```python
from build123d import *

# Parameters (mm, degrees)
F2_R     = 1.5875
F3_DEPTH = 21.717
F4_R     = 4.7625
F5_DEPTH = 9.525


with BuildPart() as f1:
    # F0 (on Front) → F1 (revolve)
    with BuildSketch(Plane.XZ):
        with BuildLine():
            Line((0, 57.6952844858), (0, 0))
            Line((0, 0), (7.62, 0))
            Line((7.62, 0), (7.62, 5.334))
            add(Edge.make_bspline(
                [(7.62, 5.334), (10.5113989407, 7.1572880683), (17.4669983954, 11.2866916591), (26.5060541886, 7.3539307829), (31.4167737961, 5.334)],
                knots=[0, 0, 0, 0, 0.4582214066, 1, 1, 1, 1], degree=3))
            Line((31.4167737961, 5.334), (31.4167737961, 37.084))
            Line((31.4167737961, 37.084), (17.8404673934, 31.6983275115))
            add(Edge.make_bspline(
                [(8.2212127745, 57.6952844858), (7.1609367505, 50.859872418), (5.223357626, 38.3686423698), (13.9081431845, 33.7772379024), (17.8404673934, 31.6983275115)],
                knots=[0, 0, 0, 0, 0.5472168907, 1, 1, 1, 1], degree=3))
            Line((8.2212127745, 57.6952844858), (0, 57.6952844858))
        make_face()
    revolve(axis=Axis((0, 0, 28.8476422429), (0, 0, 1)))

    # F2 (on face) → F3 (cut)
    with BuildSketch(Plane(origin=(0, 0, 0), x_dir=(1, 0, 0), z_dir=(0, 0, -1))):
        Circle(F2_R)
    extrude(amount=-F3_DEPTH, mode=Mode.SUBTRACT)

    # F4 (on face) → F5 (cut)
    with BuildSketch(Plane.XY.offset(57.6952844858)):
        Circle(F4_R)
    extrude(amount=-F5_DEPTH, mode=Mode.SUBTRACT)


solid = f1.part
```
Work out the finished part from the listing and answer in its coordinate system (mm). A direction names the side the tool comes from. Give positions to 0.01 mm unless a question says otherwise; leave off trailing zeros. Order: outer loops, then holes, each group sorted by start corner. A loop starts at its lowest first (then second) coordinate and runs counter-clockwise, first axis right, second up. Notation, with made-up numbers: (4.5, 5) -> (25.5, 5) arc R16 cw to (25.5, 11) -> close; hole circle Ø4 at (-6.5, 72.25). An arc over 180 degrees is marked (long way). Answer as CSV lines item,"result". Start each with the question number.
(1) Each of these flat-tipped pins is pushed along its axis until it touches: pin 1 Ø4 at (x, y) = (14.5, 15.5) entering from +Z; pin 2 Ø12 at (x, z) = (2.5, 38.5) entering from +Y; pin 3 Ø2 at (x, y) = (7.5, 5) entering from -Z. Where does it stop, or does it pass through?
(2) For a pull along X with two mould halves and no side action, classify faces 4 (the flat face through (0, 0, 21.717)), 5 (the cylindrical face through (-3.78, -2.9, 53)), 6 (the cylindrical face through (-1.65, -7.44, 2.7)), 7 (the flat face through (4, -4, 57.695)) as released by +X, released by -X, zero draft, split by the parting line, or undercut.
(3) Section A-A, the plane z = 11.5 is taken. Write down the section's boundary in (x, y) (1 decimal), plus the area to 3 significant figures.
(4) Which of the six approach directions +Z, -Z, +X, -X, +Y, -Y give full straight-line access (tool end or side, diameter ignored) to faces 1 (the cylindrical face through (-0.34, 1.55, 10.71)), 2 (the flat face through (0, 0, 48.17)), 3 (the cylindrical face through (29.966, 9.437, 21.431))?
(5) Consider line 1 along Y through (x, z) = (0, 17.5); line 2 along Z through (x, y) = (3, -1); line 3 along Y through (x, z) = (0, 55). Determine where each line is inside the solid, lowest interval first.
Entries:
1,pin 1,"z = 33.83"
1,pin 2,"y = 31.42"
1,pin 3,"z = 5.58"
2,face 4,"undercut"
2,face 5,"undercut"
2,face 6,"split by the parting line"
2,face 7,"zero draft"
3,outline,"circle Ø62.8 at (0, 0); hole circle Ø3.2 at (0, 0)"
3,area,"3,090 mm²"
4,face 1,"-Z"
4,face 2,"+Z"
4,face 3,"+Z, -Z"
5,line 1,"-31.42 to -1.59, 1.59 to 31.42"
5,line 2,"0 to 48.17"
5,line 3,"-7.81 to -4.76, 4.76 to 7.81"
